Model file for the job. Use its own axes, mm. Give positions to 0.01 mm unless a question says otherwise; leave off trailing zeros. Loops run counter-clockwise (first coordinate to the right, second up) from the corner with the lowest first, then second, coordinate; pieces in that order, holes last. Notation, with made-up numbers: M 28.5,43.25 L 46.5,43.25 A19 cw 46.5,57.25 Z; hole C -12,34.25 d6. An arc over 180 degrees is marked long. Answer in a Markdown table with one row per item.
```python
from build123d import *

# Parameters (mm, degrees)
F0_W     = 304.8
F0_H     = 101.6
F1_DEPTH = 12.7
F2_D     = 6.5278
F2_DEPTH = 16.9460333333
F2_TIP   = 1.9611489744
F3_D     = 17.4752
F3_DEPTH = 16.9418
F3_TIP   = 5.2500797448


with BuildPart() as f1:
    # F0 (on Top) → F1 (new body)
    with BuildSketch(Plane.XY):
        with Locations((152.4, 50.8)):
            Rectangle(F0_W, F0_H)
    extrude(amount=F1_DEPTH)

    # F2
    with Locations(Plane(origin=(0, 0, 0), x_dir=(1, 0, 0), z_dir=(0, 0, -1))):
        with Locations((68.58, -76.2), (68.58, -25.4), (236.22, -76.2), (236.22, -25.4)):
            Hole(F2_D / 2, depth=F2_DEPTH)
            with Locations((0, 0, -(F2_DEPTH + F2_TIP / 2))):  # 118° drill point
                Cone(0, F2_D / 2, F2_TIP, mode=Mode.SUBTRACT)

    # F3
    with Locations(Plane(origin=(0, 0, 0), x_dir=(1, 0, 0), z_dir=(0, 0, -1))):
        with Locations((152.4, -50.8)):
            Hole(F3_D / 2, depth=F3_DEPTH)
            with Locations((0, 0, -(F3_DEPTH + F3_TIP / 2))):  # 118° drill point
                Cone(0, F3_D / 2, F3_TIP, mode=Mode.SUBTRACT)


solid = f1.part
```
(1) Saw through at D-D, the plane x = 152.4. Give the cut face in (y, z), and give its area (3 significant figures).
Established:
| item | result |
|---|---|
| outline | M 0,0 L 42.06,0 L 42.06,12.7 L 0,12.7 Z; M 59.54,0 L 101.6,0 L 101.6,12.7 L 59.54,12.7 Z |
| area | 1,070 mm2 |
(2) Saw through at A-A, the plane y = 50.8. Give the cut face in (x, z).
Established:
| item | result |
|---|---|
| outline | M 0,0 L 143.66,0 L 143.66,12.7 L 0,12.7 Z; M 161.14,0 L 304.8,0 L 304.8,12.7 L 161.14,12.7 Z |
(3) Mould opens along Y. For faces 1 (the flat face through (150, 0, 6)), 2 (the cylindrical face through (234.465, 73.448, 6.439)), 3 (the flat face through (0, 50, 6)) say: pulls with the +Y half, pulls with the -Y half, needs draft (parallel to the pull), parting line crosses it, or undercut.
Established:
| item | result |
|---|---|
| face 1 | pulls with the -Y half |
| face 2 | undercut |
| face 3 | needs draft |
(4) Saw through at B-B, the plane x = 236.22. Give the cut face in (y, z).
Established:
| item | result |
|---|---|
| outline | M 0,0 L 22.14,0 L 22.14,12.7 L 0,12.7 Z; M 28.66,0 L 72.94,0 L 72.94,12.7 L 28.66,12.7 Z; M 79.46,0 L 101.6,0 L 101.6,12.7 L 79.46,12.7 Z |
(5) Wall check: L1, parallel to X at y = 25.4, z = 6.5; L2, parallel to Y at x = 236.22, z = 3; L3, parallel to Y at x = 152.4, z = 5. Give the ranges that are in metal, low to high.
Established:
| item | result |
|---|---|
| L1 | x = 0 to 65.32, 71.84 to 232.96, 239.48 to 304.8 |
| L2 | y = 0 to 22.14, 28.66 to 72.94, 79.46 to 101.6 |
| L3 | y = 0 to 42.06, 59.54 to 101.6 |
(6) Saw through at C-C, the plane y = 25.4. Give the cut face in (x, z), and give its area (3 significant figures).
Established:
| item | result |
|---|---|
| outline | M 0,0 L 65.32,0 L 65.32,12.7 L 0,12.7 Z; M 71.84,0 L 232.96,0 L 232.96,12.7 L 71.84,12.7 Z; M 239.48,0 L 304.8,0 L 304.8,12.7 L 239.48,12.7 Z |
| area | 3,710 mm2 |
